Design review of the part built by this model. Coordinates are the model's own, in mm. A direction names the side the tool comes from. Coordinates: 2 decimals unless noted, no trailing zeros. Write each loop counter-clockwise with the first axis right and the second up, starting at its lowest first coordinate (ties: lowest second). Pieces come first, ordered by that corner, then holes. Notation, with made-up numbers: M 30.5,59.5 L 86.5,59.5 A32 ccw 86.5,98.5 Z; hole C 73.5,8 d11. An arc over 180 degrees is marked long. Write each question's results on one line, items separated by ' | '. Start each with the question number.
```python
from build123d import *

# Parameters (mm, degrees)
SALIENTE_EXTRUIR1_DEPTH      = 5
SALIENTE_EXTRUIR1_DEPTH_BACK = 5
CROQUIS6_R                   = 1.75
CORTAR_EXTRUIR4_DEPTH        = 19
REDONDEO1_R                  = 5


with BuildPart() as part:
    # Croquis1 → Saliente-Extruir1 (new body, two sides)
    with BuildSketch(Plane.XY) as saliente_extruir1_sk:
        with BuildLine():
            Line((4.183300133, 8.75), (16, 8.75))
            Line((16, 8.75), (16, 15))
            Line((16, 15), (7.141428429, 15))
            ThreePointArc((7.141428429, 15), (0, 18), (-7.141428429, 15))
            Line((-7.141428429, 15), (-16, 15))
            Line((-16, 15), (-16, 0))
            Line((-16, 0), (16, 0))
            Line((16, 0), (16, 7.25))
            Line((16, 7.25), (4.183300133, 7.25))
            ThreePointArc((4.183300133, 7.25), (-4.25, 8), (4.183300133, 8.75))
        make_face()
    extrude(amount=SALIENTE_EXTRUIR1_DEPTH)
    extrude(saliente_extruir1_sk.sketch, amount=-SALIENTE_EXTRUIR1_DEPTH_BACK)

    # Croquis6 → Cortar-Extruir4 (cut, through all)
    with BuildSketch(Plane.XZ):
        with Locations((-12, 0)):
            Circle(CROQUIS6_R)
        with Locations((12, 0)):
            Circle(CROQUIS6_R)
    extrude(amount=-CORTAR_EXTRUIR4_DEPTH, mode=Mode.SUBTRACT)

    # Redondeo1
    redondeo1_edges = [part.edges().sort_by_distance(p)[0] for p in [
        (-7.141428429, 15, 0),
        (7.141428429, 15, 0),
    ]]
    fillet(redondeo1_edges, radius=REDONDEO1_R)


solid = part.part
```
Item 1: We need section C-C on x = 0. State the section outline as (y, z) points.
Item 2: We need section A-A on x = 12. State the section outline as (y, z) points, then the cut area to 4 significant figures.
Item 3: For faces 1 (the flat face through (10, 8.75, 0)), 2 (the flat face through (-14, 15, 0)), 3 (the flat face through (16, 12, 0)), list the 3-axis set-ups (+Z, -Z, +X, -X, +Y, -Y) from which the entire face can be reached by the end or side of a thin tool; tool diameter is ignored.
Item 4: We need section D-D on y = 13.75. State the section outline as (x, z) points.
Item 5: Draft analysis for pull direction Z (two halves, no side actions). For faces 4 (the flat face through (-4, 5, -5)), 5 (the cylindrical face through (13.669, 11.831, 0.526)), 6 (the flat face through (14, 15, 0)), state which applies: released by +Z, released by -Z, zero draft, split by the parting line, or undercut.
Item 6: We need section B-B on z = 0. State the section outline as (x, y) points.
Item 7: Insertion check: pin 1 Ø5.5 at (x, z) = (13.5, -2.5) entering from +Y. The pin has a flat end and moves straight along its axis. Give the tip position at first contact, or say it passes through.
Item 8: Wall thickness on L1, parallel to Z at x = 12, y = 2.5; L2, parallel to Y at x = 11, z = 2.5; L3, parallel to X at y = 2.75, z = 0.75: over which ranges is each line inside the solid? List them lowest first.
Answer:
1) outline: M 0,-5 L 3.75,-5 L 3.75,5 L 0,5 Z; M 12.25,-5 L 18,-5 L 18,5 L 12.25,5 Z
2) outline: M 0,-5 L 7.25,-5 L 7.25,-1.75 L 0,-1.75 Z; M 0,1.75 L 7.25,1.75 L 7.25,5 L 0,5 Z; M 8.75,-5 L 15,-5 L 15,-1.75 L 8.75,-1.75 Z; M 8.75,1.75 L 15,1.75 L 15,5 L 8.75,5 Z | area: 87.75 mm^2
3) face 1: +Z, -Z, +X | face 2: +Z, -Z, -X, +Y | face 3: +Z, -Z, +X, +Y, -Y
4) outline: M -16,-5 L 16,-5 L 16,5 L -16,5 Z; hole C -12,0 d3.5; hole C 12,0 d3.5
5) face 4: released by -Z | face 5: undercut | face 6: zero draft
6) outline: M -16,0 L -13.75,0 L -13.75,15 L -16,15 Z; M -10.25,0 L 10.25,0 L 10.25,7.25 L 4.18,7.25 A4.25 cw long 4.18,8.75 L 10.25,8.75 L 10.25,15 L 9,15 A5 cw 6,16 A10 ccw -6,16 A5 cw -9,15 L -10.25,15 Z; M 13.75,0 L 16,0 L 16,7.25 L 13.75,7.25 Z; M 13.75,8.75 L 16,8.75 L 16,15 L 13.75,15 Z
7) pin 1: stops at y = 15
8) L1: z = -5 to -1.75, 1.75 to 5 | L2: y = 0 to 7.25, 8.75 to 15 | L3: x = -16 to -13.58, -10.42 to 10.42, 13.58 to 16
